Autodesk Inventor part; units mm, degrees
ref_plane "YZ Plane" through (0, 0, 0) normal (1, 0, 0) x (0, 1, 0)
ref_plane "XZ Plane" through (0, 0, 0) normal (0, 1, 0) x (-1, 0, 0)
ref_plane "XY Plane" through (0, 0, 0) normal (0, 0, 1) x (1, 0, 0)
sketch "Sketch1" plane through (0, 0, 0) normal (0, 1, 0) x (-1, 0, 0)
  line L0 (0, 0) -> (-30.566, 0)
  line L1 (-30.566, 0) -> (-30.566, -53)
  line L2 (-30.566, -53) -> (0, -53)
  line L3 (0, -53) -> (0, 0)
  dimension "d0" = 30.566
  dimension "d1" = 53
extrude "Extrusion1" add sketch "Sketch1" along normal blind 2
ref_plane "Work Plane1" through (30.566, 0, -23) normal (0, 0, -1) x (-1, 0, 0)
sketch "Sketch2" plane through (30.566, 0, -23) normal (0, 0, -1) x (-1, 0, 0)
  point P0 (30.566, 0)
sketch "Sketch3" plane through (30.566, 0, -53) normal (0, 0, -1) x (-1, 0, 0)
  circle A0 centre (30.566, 0) radius 1
  circle A1 centre (30.566, 0) radius 2
  line L0 (30.566, -2) -> (15.283, 0)
  line L1 (15.283, 0) -> (28.566, 0)
  line L2 (0, 0) -> (30.566, 0)
  dimension "d5" = 2
  dimension "d6" = 4
extrude "Extrusion2" add sketch "Sketch3" against normal blind 53 contours A1 L0 | A1 L0 L1 picked at (30.3543, -1.6418)
sketch "Sketch4" plane through (30.566, 0, -53) normal (0, 0, -1) x (-1, 0, 0)
  arc A0 (29.566, 0) -> (30.566, 1) centre (30.566, 0) ccw
  circle A1 centre (30.566, 0) radius 1
  point P0 (30.566, 1)
extrude "Extrusion3" cut sketch "Sketch4" against normal blind 53
chamfer "Chamfer2" distance 2 angle 45 1 edges at (30.566, 0, -26.5)
sketch "Sketch5" plane through (0, 0, 0) normal (0, 0, 1) x (1, 0, 0)
  circle A0 centre (0, 0) radius 1
extrude "Extrusion4" add sketch "Sketch5" along normal blind 2 and the other way blind 55
chamfer "Chamfer3" distance 0.5 angle 45 1 edges at (-1, 0, 2)
chamfer "Chamfer4" distance 0.5 angle 45 1 edges at (-1, 0, -55)
equation "\"BendRadius\" = Thickness"
equation "\"BendReliefWidth\" = Thickness"
equation "\"BendReliefDepth\" = 0.5 * Thickness"
equation "\"CornerReliefSize\" = 4 * Thickness"
equation "\"MinimumRemnant\" = 2 * Thickness"
equation "\"TransitionRadius\" = BendRadius"
equation "\"JacobiRadiusSize\" = BendRadius"
equation "\"GapSize\" = Thickness"
properties part number "Part7v2"
Input: part model. Units: mm. Frame: model coordinates. A direction names the side the tool comes from. Give positions to 0.01 mm unless a question says otherwise; leave off trailing zeros. Order: outer loops, then holes, each group sorted by start corner. A loop starts at its lowest first (then second) coordinate and runs counter-clockwise, first axis right, second up. Notation, with made-up numbers: M -21,7 L 36,7 A17 ccw 36,23 Z; hole C 29.5,-30.75 d3. An arc over 180 degrees is marked long. One line per question, with ' | ' between items. Start each with the question number.
1. Section query B-B (x = 28). Return the cut outline in (y, z).
2. Section query C-C (x = 7.5). Return the cut outline in (y, z).
3. Access query for faces 1 (the face through (0, -1, -54)), 2 (the face through (0, 0, -55)), 3 (the face through (0, 1, 1)), 4 (the face through (22, 0, -26)). Directions: +Z, -Z, +X, -X, +Y, -Y. A direction counts if a zero-diameter tool reaches every point of the face in a straight line with its end or side. Return the directions, or none.
4. Material intervals for probe 1 along Z at (x, y) = (12.5, 0.1); probe 2 along Y at (x, z) = (17, -35); probe 3 along Y at (x, z) = (29.5, -39), sorted ascending. Write a range as [from, to].
5. First-contact query: pin 1 Ø1 at (x, z) = (20.5, -25) entering from -Y; pin 2 Ø1 at (x, y) = (11, 1) entering from +Z; pin 3 Ø1 at (x, y) = (6.5, 0.5) entering from -Z. Flat tips, straight axial feed; report the tip coordinate or a pass-through.
Here are the results:
1) outline: M 0,-53 L 2,-53 L 2,0 L 0,0 Z
2) outline: M -1.02,-53 L 2,-53 L 2,0 L -1.02,0 Z
3) face 1: -Z | face 2: -Z, +X, -X, +Y, -Y | face 3: +Z | face 4: +Z, -Z, +X, -Y
4) probe 1: [-53, 0] | probe 2: [0, 2] | probe 3: [0.93, 2]
5) pin 1: y = 0 | pin 2: z = 0 | pin 3: z = -53
